```python
from build123d import *

# Parameters (mm, degrees)
ESQUISSE1_R             = 2.25
ESQUISSE1_R_2           = 2.5
ESQUISSE1_R_3           = 17.5
BOSS_EXTRU_1_DEPTH      = 10
ESQUISSE2_W             = 57
ESQUISSE2_H             = 57
ENL_V_MAT_EXTRU_2_DEPTH = 5
ENL_V_MAT_EXTRU_3_DEPTH = 3
ESQUISSE5_R             = 4
ENL_V_MAT_EXTRU_4_DEPTH = 3.4


with BuildPart() as part:
    # Esquisse1 → Boss.-Extru.1 (new body)
    with BuildSketch(Plane.XY):
        with BuildLine():
            Line((5, -40), (-5, -40))
            ThreePointArc((-5, -40), (-29.748737342, -29.748737342), (-40, -5))
            Line((-40, -5), (-40, 5))
            ThreePointArc((-40, 5), (-29.748737342, 29.748737342), (-5, 40))
            Line((-5, 40), (5, 40))
            ThreePointArc((5, 40), (29.748737342, 29.748737342), (40, 5))
            Line((40, 5), (40, -5))
            ThreePointArc((40, -5), (29.748737342, -29.748737342), (5, -40))
        make_face()
        with Locations((22, 0)):
            Circle(ESQUISSE1_R, mode=Mode.SUBTRACT)
        with Locations((11, -19.052558883)):
            Circle(ESQUISSE1_R, mode=Mode.SUBTRACT)
        with Locations((-11, -19.052558883)):
            Circle(ESQUISSE1_R, mode=Mode.SUBTRACT)
        with Locations((-22, 0)):
            Circle(ESQUISSE1_R, mode=Mode.SUBTRACT)
        with Locations((-11, 19.052558883)):
            Circle(ESQUISSE1_R, mode=Mode.SUBTRACT)
        with Locations((11, 19.052558883)):
            Circle(ESQUISSE1_R, mode=Mode.SUBTRACT)
        with Locations((-23.5, 23.55)):
            Circle(ESQUISSE1_R_2, mode=Mode.SUBTRACT)
        with Locations((23.5, 23.55)):
            Circle(ESQUISSE1_R_2, mode=Mode.SUBTRACT)
        with Locations((23.5, -23.55)):
            Circle(ESQUISSE1_R_2, mode=Mode.SUBTRACT)
        with Locations((-23.5, -23.55)):
            Circle(ESQUISSE1_R_2, mode=Mode.SUBTRACT)
        Circle(ESQUISSE1_R_3, mode=Mode.SUBTRACT)
    extrude(amount=BOSS_EXTRU_1_DEPTH)

    # Esquisse2 → Enlèv. mat.-Extru.2 (cut)
    with BuildSketch(Plane(origin=(0, 0, 0), x_dir=(-1, 0, 0), z_dir=(0, 0, -1))):
        Rectangle(ESQUISSE2_W, ESQUISSE2_H)
    extrude(amount=-ENL_V_MAT_EXTRU_2_DEPTH, mode=Mode.SUBTRACT)

    # Esquisse4 → Enlèv. mat.-Extru.3 (cut)
    with BuildSketch(Plane(origin=(0, 0, 5), x_dir=(-1, 0, 0), z_dir=(0, 0, -1))):
        Polygon((-7.496491289, 21.067207559), (-10.992982578, 23.094010768), (-14.496491289, 21.079362091), (-14.503508711, 17.037910207), (-11.007017422, 15.011106999), (-7.503508711, 17.025755675), align=None)
        Polygon((14.496491289, 17.025755675), (14.503508711, 21.067207559), (11.007017422, 23.094010768), (7.503508711, 21.079362091), (7.496491289, 17.037910207), (10.992982578, 15.011106999), align=None)
        Polygon((21.992982578, -4.041451884), (25.496491289, -2.026803208), (25.503508711, 2.014648676), (22.007017422, 4.041451884), (18.503508711, 2.026803208), (18.496491289, -2.014648676), align=None)
        Polygon((7.496491289, -21.067207559), (10.992982578, -23.094010768), (14.496491289, -21.079362091), (14.503508711, -17.037910207), (11.007017422, -15.011106999), (7.503508711, -17.025755675), align=None)
        Polygon((-14.496491289, -17.025755675), (-14.503508711, -21.067207559), (-11.007017422, -23.094010768), (-7.503508711, -21.079362091), (-7.496491289, -17.037910207), (-10.992982578, -15.011106999), align=None)
        Polygon((-21.992982578, 4.041451884), (-25.496491289, 2.026803208), (-25.503508711, -2.014648676), (-22.007017422, -4.041451884), (-18.503508711, -2.026803208), (-18.496491289, 2.014648676), align=None)
    extrude(amount=-ENL_V_MAT_EXTRU_3_DEPTH, mode=Mode.SUBTRACT)

    # Esquisse5 → Enlèv. mat.-Extru.4 (cut)
    with BuildSketch(Plane.XY.offset(10)):
        with Locations((-23.5, 23.55)):
            Circle(ESQUISSE5_R)
        with Locations((-23.5, -23.55)):
            Circle(ESQUISSE5_R)
        with Locations(Location((23.5, 23.55, 0), (0, 0, 180))):
            Circle(ESQUISSE5_R)
        with Locations(Location((23.5, -23.55, 0), (0, 0, 180))):
            Circle(ESQUISSE5_R)
    extrude(amount=-ENL_V_MAT_EXTRU_4_DEPTH, mode=Mode.SUBTRACT)


solid = part.part
```
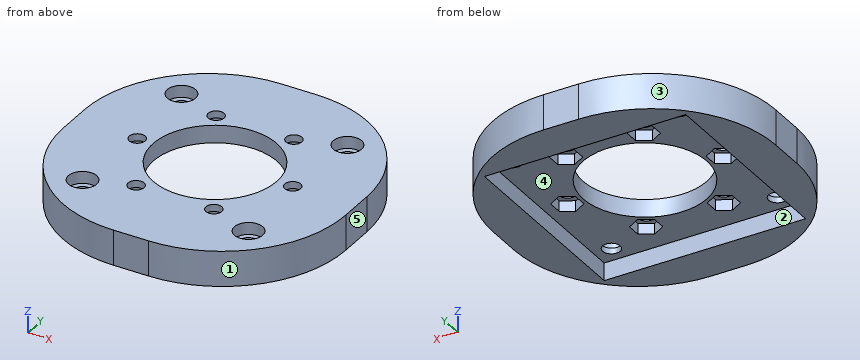
Part model, mm, in its own coordinate system. Face numbers are marked on the shaded views. A direction names the side the tool comes from. Round coordinates to 2 decimals unless told otherwise and drop trailing zeros. Write each loop counter-clockwise with the first axis right and the second up, starting at its lowest first coordinate (ties: lowest second). Pieces come first, ordered by that corner, then holes.
Item 1: Drop flat-ended pins along their axis: pin 1 Ø2.5 at (x, y) = (-22, 0) entering from -Z; pin 2 Ø1.5 at (y, z) = (18.5, 8.5) entering from +X; pin 3 Ø1 at (x, z) = (21, 6) entering from -Y; pin 4 Ø6.5 at (x, y) = (-23.5, 23.55) entering from -Z. Give the stop position or say it passes through.
Results:
pin 1: passes through
pin 2: stops at x = 37.6
pin 3: stops at y = -36.38
pin 4: stops at z = 5
Item 2: Which spindle directions (+Z, -Z, +X, -X, +Y, -Y) get a long thin tool onto all of the face, cutting with end or side? Do the marked faces 1 and 2. Say none if no direction does.
Results:
face 1: +Z, -Z, +X, -Y
face 2: -Z
Item 3: Two-plate mould, pull along Y, no slides. Class the marked faces 3, 4 and 5: +Y half, -Y half, draft (parallel to the pull), parting line (faces both ways), or undercut.
Results:
face 3: +Y half
face 4: undercut
face 5: draft
Item 4: Cut at C-C, the plane y = 13.5. Give the cut face in (x, z).
Results:
outline: (-38.95, 0) - (-28.5, 0) - (-28.5, 5) - (-11.14, 5) - (-11.14, 10) - (-38.95, 10) - close; (11.14, 5) - (28.5, 5) - (28.5, 0) - (38.95, 0) - (38.95, 10) - (11.14, 10) - close
Item 5: Cut at A-A, the plane x = 0. Give the cut face in (y, z), plus the area to 3 significant figures.
Results:
outline: (-40, 0) - (-28.5, 0) - (-28.5, 5) - (-17.5, 5) - (-17.5, 10) - (-40, 10) - close; (17.5, 5) - (28.5, 5) - (28.5, 0) - (40, 0) - (40, 10) - (17.5, 10) - close
area: 340 mm2
Item 6: Probe L1, parallel to X at y = 0, z = 6.6; L2, parallel to Y at x = 0, z = 8.9; L3, parallel to Y at x = 23.5, z = 8.6. List the from-to ranges inside material, lowest first.
Results:
L1: x = -40 to -25.5, -18.5 to -17.5, 17.5 to 18.5, 25.5 to 40
L2: y = -40 to -17.5, 17.5 to 40
L3: y = -34.71 to -27.55, -19.55 to -1.68, 1.68 to 19.55, 27.55 to 34.71
Item 7: Cut at B-B, the plane z = 3.25. Give the cut face in (x, y), plus the area to 3 significant figures.
Results:
outline: (-40, -5) arc R35 ccw to (-5, -40) - (5, -40) arc R35 ccw to (40, -5) - (40, 5) arc R35 ccw to (5, 40) - (-5, 40) arc R35 ccw to (-40, 5) - close; hole (-28.5, -28.5) - (28.5, -28.5) - (28.5, 28.5) - (-28.5, 28.5) - close
area: 2,100 mm2
